from build123d import *

# Parameters (mm, degrees)
BOSS_EXTRUDE1_DEPTH = 0.8
FILLET1_R           = 2
FILLET2_R           = 5
SKETCH2_R           = 1.2
CUT_EXTRUDE1_DEPTH  = 23.249719099
SKETCH3_R           = 1.2
CUT_EXTRUDE2_DEPTH  = 23.249719099


with BuildPart() as part:
    # Sketch1 → Boss-Extrude1 (new, symmetric)
    with BuildSketch(Plane(origin=(0, 0, 0), x_dir=(1, 0, 0), z_dir=(0, 1, 0))):
        with BuildLine():
            Line((11.716387939, 7), (-8.827016654, 7))
            ThreePointArc((-8.827016654, 7), (-20.7, 0), (-8.827016654, -7))
            Line((-8.827016654, -7), (11.716387939, -7))
            Line((11.716387939, -7), (11.716387939, 7))
        make_face()
    extrude(amount=BOSS_EXTRUDE1_DEPTH, both=True)

    # Fillet1
    fillet1_edges = [part.edges().sort_by_distance(p)[0] for p in [
        (11.716387939, 0, 7),
        (11.716387939, 0, -7),
    ]]
    fillet(fillet1_edges, radius=FILLET1_R)

    # Fillet2
    fillet2_edges = [part.edges().sort_by_distance(p)[0] for p in [
        (-8.827016654, 0, 7),
        (-8.827016654, 0, -7),
    ]]
    fillet(fillet2_edges, radius=FILLET2_R)

    # Sketch2 → Cut-Extrude1 (cut, through all)
    with BuildSketch(Plane(origin=(0, 0.8, 0), x_dir=(1, 0, 0), z_dir=(0, 1, 0))):
        with Locations(Location((-8.2, 0, 0), (0, 0, 270))):
            Circle(SKETCH2_R)
        with Locations(Location((-12.7, 4.5, 0), (0, 0, 270))):
            Circle(SKETCH2_R)
        with Locations(Location((-17.2, 0, 0), (0, 0, 270))):
            Circle(SKETCH2_R)
        with Locations(Location((-12.7, -4.5, 0), (0, 0, 270))):
            Circle(SKETCH2_R)
        with Locations(Location((-12.7, 0, 0), (0, 0, 270))):
            Circle(SKETCH2_R)
    extrude(amount=-CUT_EXTRUDE1_DEPTH, mode=Mode.SUBTRACT)

    # Sketch3 → Cut-Extrude2 (cut, through all)
    with BuildSketch(Plane(origin=(0, 0.8, 0), x_dir=(1, 0, 0), z_dir=(0, 1, 0))):
        with Locations(Location((9.121387939, 4.25, 0), (0, 0, 270))):
            Circle(SKETCH3_R)
        with Locations(Location((9.121387939, -4.25, 0), (0, 0, 270))):
            Circle(SKETCH3_R)
        with Locations(Location((6.871387939, 0, 0), (0, 0, 270))):
            Circle(SKETCH3_R)
    extrude(amount=-CUT_EXTRUDE2_DEPTH, mode=Mode.SUBTRACT)


solid = part.part
Can you work these out from the model? Positions are in its coordinate system, mm. A direction names the side the tool comes from. Coordinates: 2 decimals unless noted, no trailing zeros. Write each loop counter-clockwise with the first axis right and the second up, starting at its lowest first coordinate (ties: lowest second). Pieces come first, ordered by that corner, then holes.
Q1. Imagine slicing it at A-A, the plane x = -8.2. List the corners of the cut face in (y, z) for me.
Results found:
outline: (-0.8, -7.03) - (0.8, -7.03) - (0.8, -1.2) - (-0.8, -1.2) - close; (-0.8, 1.2) - (0.8, 1.2) - (0.8, 7.03) - (-0.8, 7.03) - close
Q2. For P1, Ø2, axis at x = 6.87, z = 0, coming from the -Y side; P2, Ø0.8, axis at x = 1.5, y = 0.5, coming from the +Z side, each with a flat end and sliding along its axis, tell me the tip position at first contact or that it passes through.
Results found:
P1: passes through
P2: stops at z = 7
Q3. Imagine slicing it at C-C, the plane y = 0.25. Count the separate pieces of the cut face and the enclosed holes in it, plus the area to 3 significant figures.
Results found:
separate pieces: 1
enclosed holes: 8
area: 410 mm2
Q4. Imagine slicing it at D-D, the plane x = -12. List the corners of the cut face in (y, z) for me.
Results found:
outline: (-0.8, -7.97) - (0.8, -7.97) - (0.8, -5.47) - (-0.8, -5.47) - close; (-0.8, -3.53) - (0.8, -3.53) - (0.8, -0.97) - (-0.8, -0.97) - close; (-0.8, 0.97) - (0.8, 0.97) - (0.8, 3.53) - (-0.8, 3.53) - close; (-0.8, 5.47) - (0.8, 5.47) - (0.8, 7.97) - (-0.8, 7.97) - close
Q5. If we mould it in two halves opening along Z, with no side actions, what happens to faces 1 (the face through (11.716, 0, 0)), 2 (the face through (11.146, -0.011, 6.399)), 3 (the face through (9.932, 0.011, 3.366)), 4 (the face through (11.115, -0.011, -6.43))? For each: +Z half, -Z half, draft (parallel to the pull), parting line (faces both ways), or undercut.
Results found:
face 1: draft
face 2: +Z half
face 3: undercut
face 4: -Z half
Q6. Imagine slicing it at B-B, the plane z = -4.5. List the corners of the cut face in (x, y) for me, plus the area to 3 significant figures.
Results found:
outline: (-19.31, -0.8) - (-13.9, -0.8) - (-13.9, 0.8) - (-19.31, 0.8) - close; (-11.5, -0.8) - (7.95, -0.8) - (7.95, 0.8) - (-11.5, 0.8) - close; (10.3, -0.8) - (11.72, -0.8) - (11.72, 0.8) - (10.3, 0.8) - close
area: 42.1 mm2
Q7. Which directions (+Z, -Z, +X, -X, +Y, -Y) give clear straight access to the entire face, cutting with the end or side of a thin tool? Please do faces 5 (the face through (-5, 0.8, 0)), 6 (the face through (1, 0, -7)), 7 (the face through (1, 0, 7)).
Results found:
face 5: +Z, -Z, +X, -X, +Y
face 6: -Z, +X, +Y, -Y
face 7: +Z, +X, +Y, -Y
Q8. Please list where these lines run through material, in increasing order: L1, parallel to X at y = 0.35, z = 0; L2, parallel to X at y = -0.4, z = 5 (3 decimals); L3, parallel to Z at x = -12, y = 0.6.
Results found:
L1: x = -20.7 to -18.4, -16 to -13.9, -11.5 to -9.4, -7 to 5.67, 8.07 to 11.72
L2: x = -18.945 to -13.791, -11.609 to 8.185, 10.058 to 11.716
L3: z = -7.97 to -5.47, -3.53 to -0.97, 0.97 to 3.53, 5.47 to 7.97
